```python
from build123d import *

# Parameters (mm, degrees)
BOSS_EXTRUDE1_DEPTH = 1.524


with BuildPart() as part:
    # Sketch1 → Boss-Extrude1 (new body)
    with BuildSketch(Plane.XY):
        with BuildLine():
            Line((37.704296416, -31.705702494), (32.621666071, -35.245462588))
            Line((32.621666071, -35.245462588), (33.493939306, -36.4982372))
            Line((33.493939306, -36.4982372), (38.576569651, -32.957484201))
            ThreePointArc((38.576569651, -32.957484201), (39.742986246, -34.371130843), (39.316039794, -36.153444291))
            ThreePointArc((39.316039794, -36.153444291), (35.743862713, -41.392315435), (33.736249861, -47.406940162))
            ThreePointArc((33.736249861, -47.406940162), (33.736605397, -47.436618983), (33.736723912, -47.466299698))
            ThreePointArc((33.736723912, -47.466299698), (31.060825363, -50.029100651), (29.678991539, -53.46696584))
            ThreePointArc((29.678991539, -53.46696584), (27.115500093, -51.083388449), (26.30925741, -47.677085129))
            ThreePointArc((26.30925741, -47.677085129), (24.451153983, -45.627042683), (21.740362101, -46.180964831))
            ThreePointArc((21.740362101, -46.180964831), (20.76513964, -49.206145699), (18.541417724, -51.477233316))
            ThreePointArc((18.541417724, -51.477233316), (19.716696181, -49.619411518), (19.289312359, -47.462996819))
            ThreePointArc((19.289312359, -47.462996819), (14.95515305, -49.204688548), (10.437184098, -50.390598976))
            ThreePointArc((10.437184098, -50.390598976), (9.740523804, -52.101024231), (8.47892764, -53.449825638))
            ThreePointArc((8.47892764, -53.449825638), (8.977567303, -52.098435339), (8.892067822, -50.66052467))
            ThreePointArc((8.892067822, -50.66052467), (3.246101629, -51.089737509), (-2.399729403, -50.658750414))
            ThreePointArc((-2.399729403, -50.658750414), (-4.344989088, -52.336657488), (-6.594422726, -53.577405529))
            ThreePointArc((-6.594422726, -53.577405529), (-5.427176524, -52.043650888), (-4.956013668, -50.174728054))
            ThreePointArc((-4.956013668, -50.174728054), (-12.354481608, -47.665032068), (-19.067256704, -43.668214296))
            ThreePointArc((-19.067256704, -43.668214296), (-20.685168003, -44.086118721), (-22.356101471, -44.069919276))
            ThreePointArc((-22.356101471, -44.069919276), (-21.34731349, -43.406825821), (-20.564738203, -42.48762941))
            ThreePointArc((-20.564738203, -42.48762941), (-24.363722181, -38.849120016), (-27.612631699, -34.712017549))
            ThreePointArc((-27.612631699, -34.712017549), (-30.00052566, -34.336897034), (-32.065024234, -33.079678433))
            ThreePointArc((-32.065024234, -33.079678433), (-30.436493757, -33.12678938), (-28.850067174, -32.755869369))
            ThreePointArc((-28.850067174, -32.755869369), (-29.339652087, -31.900308765), (-29.806440493, -31.032100312))
            ThreePointArc((-29.806440493, -31.032100312), (-32.582725704, -24.1759064), (-34.009509312, -16.917845842))
            ThreePointArc((-34.009509312, -16.917845842), (-36.514142372, -16.032312472), (-38.402522283, -14.16378968))
            ThreePointArc((-38.402522283, -14.16378968), (-36.306570998, -14.636822999), (-34.162260401, -14.773586932))
            ThreePointArc((-34.162260401, -14.773586932), (-34.180156343, -14.293685665), (-34.192120126, -13.813599883))
            ThreePointArc((-34.192120126, -13.813599883), (-34.621527317, -7.717500789), (-34.994580248, -1.617693725))
            ThreePointArc((-34.994580248, -1.617693725), (-38.013814487, -0.220962087), (-39.79584853, 2.588128395))
            ThreePointArc((-39.79584853, 2.588128395), (-37.649043689, 1.2668877), (-35.139082483, 1.033343809))
            ThreePointArc((-35.139082483, 1.033343809), (-35.751631039, 15.891841194), (-36.02990482, 30.760355712))
            ThreePointArc((-36.02990482, 30.760355712), (-38.387515912, 33.373438153), (-39.306278852, 36.770849603))
            ThreePointArc((-39.306278852, 36.770849603), (-37.931736179, 34.774118143), (-36.043826919, 33.253558144))
            ThreePointArc((-36.043826919, 33.253558144), (-36.047258198, 36.901464596), (-36.030566217, 40.549334472))
            ThreePointArc((-36.030566217, 40.549334472), (-35.002266591, 47.029894856), (-34.571956243, 53.577405529))
            ThreePointArc((-34.571956243, 53.577405529), (-33.341283224, 38.509314077), (-33.703754569, 23.395394975))
            ThreePointArc((-33.703754569, 23.395394975), (-32.823671192, 4.023096585), (-31.30799989, -15.309860564))
            ThreePointArc((-31.30799989, -15.309860564), (-13.310528761, -43.455618792), (20.06424012, -41.96649978))
            ThreePointArc((20.06424012, -41.96649978), (21.243050758, -40.73566209), (21.723238049, -39.10043241))
            ThreePointArc((21.723238049, -39.10043241), (18.8276625, -36.637371423), (15.353729803, -35.093733252))
            ThreePointArc((15.353729803, -35.093733252), (21.571557105, -34.969630573), (27.700749295, -33.916169174))
            ThreePointArc((27.700749295, -33.916169174), (29.941679247, -32.068657032), (31.293105646, -29.497914951))
            ThreePointArc((31.293105646, -29.497914951), (32.948684374, -29.840980808), (34.616890834, -30.116157682))
            ThreePointArc((34.616890834, -30.116157682), (36.353174649, -30.536876005), (37.704296416, -31.705702494))
        make_face()
    extrude(amount=BOSS_EXTRUDE1_DEPTH)


solid = part.part
```
Verification items for the finished model (mm, model axes). A direction names the side the tool comes from. Give positions to 0.01 mm unless a question says otherwise; leave off trailing zeros. Write each loop counter-clockwise with the first axis right and the second up, starting at its lowest first coordinate (ties: lowest second). Pieces come first, ordered by that corner, then holes. Notation, with made-up numbers: (22, -12) - (80, -12) arc R8 cw to (80, 2) - close; hole circle Ø6 at (66, 41.25). An arc over 180 degrees is marked (long way). Put each result on its own line as item: value.
Q1. Section check A-A on y = -26.5. Record the cut outline in (x, z), and give its area (3 significant figures).
Result:
outline: (-31.81, 0) - (-28.83, 0) - (-28.83, 1.52) - (-31.81, 1.52) - close
area: 4.54 mm2
Q2. Scan lines: probe 1 along Y at (x, z) = (-29, 1.05); probe 2 along Y at (x, z) = (20, 0.55); probe 3 along X at (y, z) = (-37, 1.2). Record each from-to range of solid material in increasing order. Write a range as from..to.
Result:
probe 1: -34.61..-32.81, -32.5..-26.08
probe 2: -50.24..-42.01, -37.47..-35.09
probe 3: -25.93..-21.97, 19.37..38.59
Q3. Section check B-B on x = 6. Record the cut outline in (y, z), and give its area (3 significant figures).
Result:
outline: (-50.99, 0) - (-46.98, 0) - (-46.98, 1.52) - (-50.99, 1.52) - close
area: 6.10 mm2
Q4. Mould release check, pull along Y, two halves, no side actions. Record for faces 6 (the face through (29.916, -32.1, 0.751)), 7 (the face through (35.784, -41.313, 0.751)), 8 (the face through (36, -34.75, 0.75)): released by +Y, released by -Y, zero draft, split by the parting line, or undercut.
Result:
face 6: released by +Y
face 7: released by -Y
face 8: undercut
Q5. Set-up check for faces 1 (the face through (-3, -47, 1.524)), 2 (the face through (20.788, -49.168, 0.751)), 3 (the face through (-38.364, 33.33, 0.751)), 4 (the face through (35.2, -33.45, 0.75)), 5 (the face through (-32.84, 4.29, 0.75)): record each of +Z, -Z, +X, -X, +Y, -Y from which the full face is reachable in a straight line by a thin tool's end or side.
Result:
face 1: +Z, +X, -X, +Y, -Y
face 2: +Z, -Z, -Y
face 3: +Z, -Z, -X
face 4: +Z, -Z
face 5: +Z, -Z, +X
Q6. Depth check by flat-ended pin: P1, Ø6, axis at x = -30, y = 6, coming from the +Z side. Enter the tip coordinate at first touch or a pass-through.
Result:
P1: z = 1.52
